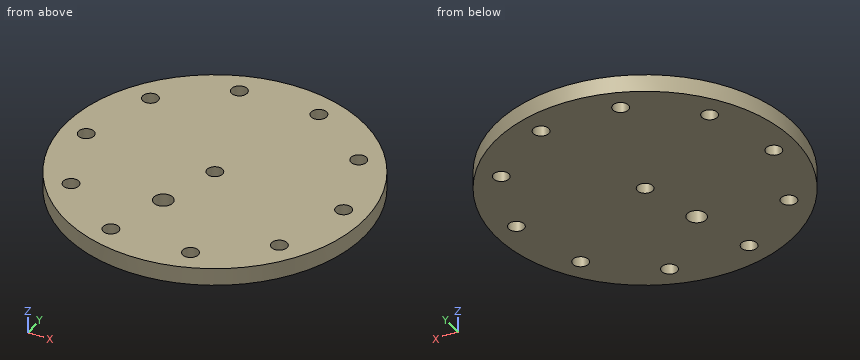
```python
from build123d import *

# Parameters (mm, degrees)
F0_R            = 76.2
F1_DEPTH        = 8.89
F2_R            = 3.937
F3_DEPTH        = 25.4
F4_R            = 4.826
F5_DEPTH        = 25.4
F6_R            = 3.9624
F7_DEPTH        = 25.4
F7_COPIES_COUNT = 10


# Not quite as in the source:
# - a pattern or mirror of a feature is missing from the dataset's text; its kind, count and spacing are read off the source's solid


with BuildPart() as f1:
    # F0 (on Top) → F1 (new body)
    with BuildSketch(Plane.XY):
        Circle(F0_R)
    extrude(amount=F1_DEPTH)

    # F2 (on face) → F3 (cut)
    with BuildSketch(Plane.XY.offset(8.89)):
        Circle(F2_R)
    extrude(amount=-F3_DEPTH, mode=Mode.SUBTRACT)

    # F4 (on face) → F5 (cut)
    with BuildSketch(Plane.XY.offset(8.89)):
        with Locations((-9.46404, -30.48)):
            Circle(F4_R)
    extrude(amount=-F5_DEPTH, mode=Mode.SUBTRACT)

    # F6 (on face) → F7 (cut)
    with BuildSketch(Plane.XY.offset(8.89)):
        with Locations((-19.085301976, -61.4663509693)):
            Circle(F6_R)
    f7 = extrude(amount=-F7_DEPTH, mode=Mode.SUBTRACT)

    # F7_copies: F7 ×10 about axis
    f7_copies_axis = Axis((0, 0, 0), (0, 0, 1))
    for i in range(1, F7_COPIES_COUNT):
        add(f7.rotate(f7_copies_axis, i * 360 / F7_COPIES_COUNT), mode=Mode.SUBTRACT)


solid = f1.part
```
Model file for the job. Use its own axes, mm. Coordinates: 2 decimals unless noted, no trailing zeros. Order: outer loops, then holes, each group sorted by start corner. A loop starts at its lowest first (then second) coordinate and runs counter-clockwise, first axis right, second up. Notation, with made-up numbers: (77.5, 35) - (125.5, 35) arc R23 cw to (125.5, 58) - close; hole circle Ø8 at (23, 18.25). An arc over 180 degrees is marked (long way). Return JSON: item names as keys, results as strings. Group by question number.
1) Saw through at D-D, the plane y = -30.48. Write the cut outline in (x, z).
2) Saw through at C-C, the plane z = 6.25. Count the separate pieces of the cut face and the enclosed holes in it, plus the area to 3 significant figures.
3) Saw through at B-B, the plane y = 0. Write the cut outline in (x, z), plus the area to 3 significant figures.
4) Flat gauge pins, fed straight in: P1, Ø2, axis at y = 16, z = 7.5, coming from the -X side; P2, Ø1.5, axis at x = 49, z = 5, coming from the -Y side; P3, Ø6.5, axis at x = 20.69, y = -60.95, coming from the +Z side. Where does each tip first touch, or does it go through?
5) Saw through at A-A, the plane x = 0. Write the cut outline in (y, z), plus the area to 3 significant figures.
6) Probe line 1 (X direction, y = 37, z = 8); line 2 (Y direction, x = 0, z = 4.5); line 3 (X direction, y = -38, z = 7.5). List the from-to ranges inside material, lowest first. Write a range as from..to.
Values found:
{
 "1": {"outline": "(-69.84, 0) - (-14.29, 0) - (-14.29, 8.89) - (-69.84, 8.89) - close; (-4.64, 0) - (69.84, 0) - (69.84, 8.89) - (-4.64, 8.89) - close"},
 "2": {"separate pieces": "1", "enclosed holes": "12", "area": "17,600 mm²"},
 "3": {"outline": "(-76.2, 0) - (-68.23, 0) - (-68.23, 8.89) - (-76.2, 8.89) - close; (-60.48, 0) - (-3.94, 0) - (-3.94, 8.89) - (-60.48, 8.89) - close; (3.94, 0) - (60.48, 0) - (60.48, 8.89) - (3.94, 8.89) - close; (68.23, 0) - (76.2, 0) - (76.2, 8.89) - (68.23, 8.89) - close", "area": "1,150 mm²"},
 "4": {"P1": "stops at x = -74.71", "P2": "stops at y = -58.98", "P3": "passes through"},
 "5": {"outline": "(-76.2, 0) - (-3.94, 0) - (-3.94, 8.89) - (-76.2, 8.89) - close; (3.94, 0) - (76.2, 0) - (76.2, 8.89) - (3.94, 8.89) - close", "area": "1,280 mm²"},
 "6": {"line 1": "x = -66.61..-56.52, -48.6..47.91, 55.23..66.61", "line 2": "y = -76.2..-3.94, 3.94..76.2", "line 3": "x = -66.05..-55.5, -47.64..48.69, 56.43..66.05"}
}
